```python
from build123d import *

# Parameters (mm, degrees)
EXTRUDE2_DEPTH = 3
SKETCH3_W      = 40
SKETCH3_H      = 3
EXTRUDE3_DEPTH = 39
SKETCH4_R      = 2
EXTRUDE4_DEPTH = 73.752827534


with BuildPart() as part:
    # Sketch1 → Extrude2 (new body)
    with BuildSketch(Plane(origin=(0, 0, 0), x_dir=(1, 0, 0), z_dir=(0, 1, 0))):
        with BuildLine():
            Line((0, 0), (40, 0))
            Line((40, 0), (40, 25))
            ThreePointArc((40, 25), (21.5, 46.5), (0, 28))
            Line((0, 28), (0, 0))
        make_face()
        with BuildLine():
            Line((26, 35.5), (26, 20.5))
            ThreePointArc((26, 20.5), (20, 14.5), (14, 20.5))
            Line((14, 20.5), (14, 35.5))
            ThreePointArc((14, 35.5), (20, 41.5), (26, 35.5))
        make_face(mode=Mode.SUBTRACT)
    extrude(amount=EXTRUDE2_DEPTH)

    # Sketch3 → Extrude3 (add)
    with BuildSketch(Plane.XZ):
        with Locations((20, -1.5)):
            Rectangle(SKETCH3_W, SKETCH3_H)
    extrude(amount=EXTRUDE3_DEPTH)

    # Sketch4 → Extrude4 (cut, through all)
    with BuildSketch(Plane.XY):
        with Locations((34.25, -7)):
            Circle(SKETCH4_R)
        with Locations((5.75, -7)):
            Circle(SKETCH4_R)
        with Locations((5.75, -29.5)):
            Circle(SKETCH4_R)
        with Locations((34.25, -29.5)):
            Circle(SKETCH4_R)
    extrude(amount=-EXTRUDE4_DEPTH, mode=Mode.SUBTRACT)


solid = part.part
```
For this review, take the finished solid that the model builds, in its own axes (mm). A direction names the side the tool comes from. Give positions to 0.01 mm unless a question says otherwise; leave off trailing zeros. Order: outer loops, then holes, each group sorted by start corner. A loop starts at its lowest first (then second) coordinate and runs counter-clockwise, first axis right, second up.
1) Wall thickness on line 1 (Y direction, x = 34, z = -1); line 2 (X direction, y = -29, z = -2); line 3 (Z direction, x = 9, y = -8.5): over which ranges is each line inside the solid? List them lowest first.
2) Take a section at A-A (z = -26.5). Give the boundary of the cut face in (x, y).
3) The part is to be moulded in two halves that separate along Z. For faces 1 (the face through (20, -19, -3)), 2 (the face through (20.1, 1.5, -14.5)), 3 (the face through (5.316, -31.452, -1.479)), say which applies: released by +Z, released by -Z, zero draft, split by the parting line, or undercut.
4) For faces 4 (the face through (24, 0, -15)), 5 (the face through (3.752, -6.912, -1.479)), 6 (the face through (19.9, 1.5, -41.5)), 7 (the face through (40, -10, -2)), list the 3-axis set-ups (+Z, -Z, +X, -X, +Y, -Y) from which the entire face can be reached by the end or side of a thin tool; tool diameter is ignored.
5) Insertion check: pin 1 (1.5 mm diameter, centred on y = 2, z = -30, fed in from +X); pin 2 (1.5 mm diameter, centred on x = 35.5, y = -23, fed in from -Z); pin 3 (12.5 mm diameter, centred on y = -16, z = -8.5, fed in from +X). Each pin has a flat end and moves straight along its axis. Give the tip position at first contact, or say it passes through.
6) Take a section at D-D (x = 6). Give the boundary of the cut face in (y, z), then the cut area to 3 significant figures.
7) Take a section at C-C (x = 20). Give the boundary of the cut face in (y, z), then the cut area to 3 significant figures.
8) Take a section at B-B (y = -29.5). Give the boundary of the cut face in (x, z).
Derived:
1. line 1: y = -39 to -31.48, -27.52 to -8.98, -5.02 to 3
1. line 2: x = 0 to 3.81, 7.69 to 32.31, 36.19 to 40
1. line 3: z = -3 to 0
2. outline: (0, 0) - (14, 0) - (14, 3) - (0, 3) - close; (26, 0) - (40.06, 0) - (40.06, 3) - (26, 3) - close
3. face 1: released by -Z
3. face 2: undercut
3. face 3: zero draft
4. face 4: -Z, +X, -X, -Y
4. face 5: +Z, -Z
4. face 6: +Y, -Y
4. face 7: +Z, +X, +Y, -Y
5. pin 1: stops at x = 39.87
5. pin 2: stops at z = -3
5. pin 3: stops at x = 40
6. outline: (-39, -3) - (-31.48, -3) - (-31.48, 0) - (-39, 0) - close; (-27.52, -3) - (-8.98, -3) - (-8.98, 0) - (-27.52, 0) - close; (-5.02, -3) - (0, -3) - (0, -40.86) - (3, -40.86) - (3, 0) - (-5.02, 0) - close
6. area: 216 mm2
7. outline: (-39, -3) - (0, -3) - (0, -14.5) - (3, -14.5) - (3, 0) - (-39, 0) - close; (0, -46.56) - (3, -46.56) - (3, -41.5) - (0, -41.5) - close
7. area: 176 mm2
8. outline: (0, -3) - (3.75, -3) - (3.75, 0) - (0, 0) - close; (7.75, -3) - (32.25, -3) - (32.25, 0) - (7.75, 0) - close; (36.25, -3) - (40, -3) - (40, 0) - (36.25, 0) - close
